from build123d import *

# Parameters (mm, degrees)
SKETCH1_R               = 12.5
BOSS_EXTRUDE1_DEPTH     = 100
CUT_EXTRUDE1_DEPTH      = 80
CHAMFER2_SIZE           = 7.5
CUT_EXTRUDE2_DEPTH      = 288.054001888
CUT_EXTRUDE2_DEPTH_BACK = 288.054001888


with BuildPart() as part:
    # Sketch1 → Boss-Extrude1 (new, symmetric)
    with BuildSketch(Plane(origin=(0, 0, 0), x_dir=(0, 0, -1), z_dir=(1, 0, 0))):
        with BuildLine():
            Line((-100, 0), (-100, -180))
            Line((-100, -180), (100, -180))
            Line((100, -180), (100, 0))
            ThreePointArc((100, 0), (0, 100), (-100, 0))
        make_face()
        Circle(SKETCH1_R, mode=Mode.SUBTRACT)
    extrude(amount=BOSS_EXTRUDE1_DEPTH, both=True)

    # Sketch2 → Cut-Revolve1 (revolve, cut)
    with BuildSketch(Plane(origin=(0, 0, 0), x_dir=(0, 0, -1), z_dir=(1, 0, 0)), mode=Mode.PRIVATE) as cut_revolve1_sk:
        Polygon((100, -180), (100, -150), (150, -90.41232037), (150, -180), align=None)
    revolve(cut_revolve1_sk.sketch.rotate(Axis((0, 100, 0), (0, -1, 0)), 180), axis=Axis((0, 100, 0), (0, -1, 0)), mode=Mode.SUBTRACT)

    # Sketch3 → Cut-Extrude1 (cut, symmetric)
    with BuildSketch(Plane(origin=(0, 0, 0), x_dir=(0, 0, -1), z_dir=(1, 0, 0))):
        with BuildLine():
            Line((-100, 0), (-100, -105))
            Line((-100, -105), (100, -105))
            Line((100, -105), (100, 0))
            ThreePointArc((100, 0), (0, 100), (-100, 0))
        make_face()
    extrude(amount=CUT_EXTRUDE1_DEPTH, both=True, mode=Mode.SUBTRACT)

    # Chamfer2
    chamfer2_edges = [part.edges().sort_by_distance(p)[0] for p in [
        (100, -50.317974947, -100),
        (100, -50.317974947, 100),
        (100, 100, 0),
        (-100, -50.317974947, -100),
        (-100, -50.317974947, 100),
        (-100, 100, 0),
    ]]
    chamfer(chamfer2_edges, length=CHAMFER2_SIZE)

    # Sketch4 → Cut-Extrude2 (cut, two sides: drawn at the far end of the back side and taken through both)
    with BuildSketch(Plane.XY.offset(100).offset(-CUT_EXTRUDE2_DEPTH_BACK)):
        with BuildLine():
            Line((-80, -105), (80, -105))
            ThreePointArc((80, -105), (0, -135.5572809), (-80, -105))
        make_face()
    extrude(amount=CUT_EXTRUDE2_DEPTH + CUT_EXTRUDE2_DEPTH_BACK, mode=Mode.SUBTRACT)


solid = part.part
Read the model definition and answer for the solid it produces. Units are mm, in the model's axes. A direction names the side the tool comes from. Give positions to 0.01 mm unless a question says otherwise; leave off trailing zeros. Loops run counter-clockwise (first coordinate to the right, second up) from the corner with the lowest first, then second, coordinate; pieces in that order, holes last. Notation, with made-up numbers: M -5.5,48 L 41.5,48 A29 cw 41.5,84 Z; hole C 48,-18 d7. An arc over 180 degrees is marked long. Write each question's results on one line, items separated by ' | '.
1. Given pin 1 (8 mm diameter, centred on x = 44.5, y = -125.5, fed in from +Z); pin 2 (1.5 mm diameter, centred on x = 67.5, z = 33.5, fed in from +Y); pin 3 (12 mm diameter, centred on x = 63.5, z = 12, fed in from +Y); pin 4 (2 mm diameter, centred on x = 75, z = 21.5, fed in from +Y), each flat-ended and moving along its own axis, determine where each tip first touches the part or whether it passes through.
Values:
pin 1: stops at z = 100 | pin 2: stops at y = -114.26 | pin 3: stops at y = -113.38 | pin 4: stops at y = -108.42
2. The mould has two halves that part along Y. Classify faces 4 (the face through (89.86, 3.755, -11.923)), 5 (the face through (1, -180, 1)), 6 (the face through (1.23, -135.55, -1.4)), 7 (the face through (-96.2, -54.2, -96.3)): pulls with the +Y half, pulls with the -Y half, needs draft (parallel to the pull), parting line crosses it, or undercut.
Values:
face 4: undercut | face 5: pulls with the -Y half | face 6: pulls with the +Y half | face 7: needs draft
3. Section A-A on y = -57 is taken. Give the vertices of the cut face in (x, z), plus the area to 3 significant figures.
Values:
outline: M -100,-92.5 L -92.5,-100 L -80,-100 L -80,100 L -92.5,100 L -100,92.5 Z; M 80,-100 L 92.5,-100 L 100,-92.5 L 100,92.5 L 92.5,100 L 80,100 Z | area: 7,890 mm^2
4. A tool of negligible diameter and unlimited length cuts with its end or side. For faces 1 (the face through (80, -24, 1)), 2 (the face through (100, -27, 1)), 3 (the face through (-30.04, -164.79, 95.38)), from which of +Z, -Z, +X, -X, +Y, -Y can it reach the whole face along a straight path? Write none if from no direction.
Values:
face 1: +Z, -Z, +Y | face 2: +Z, -Z, +X, +Y, -Y | face 3: -Y
5. Straight lines are drawn through the part: line 1 (Y direction, x = -92, z = 0); line 2 (X direction, y = -17, z = -81.5); line 3 (X direction, y = -118.5, z = 62). For each, find the intervals that lie inside material, in ascending order. Write a range as [from, to].
Values:
line 1: y = [-180, -12.5], [12.5, 100] | line 2: x = [-100, -80], [80, 100] | line 3: x = [-100, -61.67], [61.67, 100]
